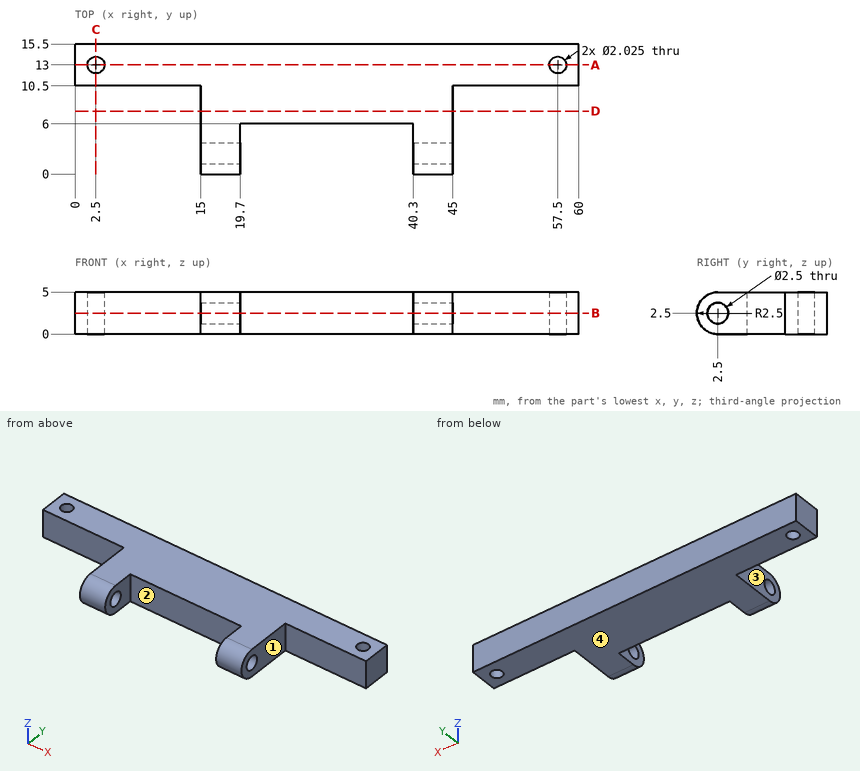
Could you check a few things on this drawing? It's one solid part, dimensions in mm from its lowest x, y, z. A direction names the side the tool comes from. Coordinates: 2 decimals unless noted, no trailing zeros. Order: outer loops, then holes, each group sorted by start corner. A loop starts at its lowest first (then second) coordinate and runs counter-clockwise, first axis right, second up.
1. If we section it at B-B (z = 2.5): Give the number of separate pieces and of enclosed holes in the cut face.
2. If we section it at A-A (y = 13): Please give me the cut outline in (x, z), then the cut area to 3 significant figures.
3. I'm going to push flat-ended pins straight in: pin 1 (3 mm diameter, centred on y = 7.5, z = 2.5, fed in from +X); pin 2 (3 mm diameter, centred on y = 8, z = 3, fed in from -X); pin 3 (1.5 mm diameter, centred on x = 10, z = 3, fed in from -Y); pin 4 (2.5 mm diameter, centred on x = 57.5, y = 13, fed in from +Z). Where does each tip first touch, or does it pass through?
4. For the marked faces 1, 2, 3 and 4, which set-ups out of +Z, -Z, +X, -X, +Y, -Y let a thin tool reach every point of the face, with its end or its side?
5. If we section it at D-D (y = 7.5): Please give me the cut outline in (x, z).
6. I need wall thicknesses on line 1 (X direction, y = 13, z = 1.25); line 2 (X direction, y = 5.5, z = 2.1); line 3 (Y direction, x = 42.55, z = 2.5). Which ranges of each line are inside material? Lowest first, please.
7. If we section it at C-C (x = 2.5): Please give me the cut outline in (y, z), then the cut area to 3 significant figures.
Entries:
1. separate pieces: 3
1. enclosed holes: 2
2. outline: (0, 0) - (1.49, 0) - (1.49, 5) - (0, 5) - close; (3.51, 0) - (56.49, 0) - (56.49, 5) - (3.51, 5) - close; (58.51, 0) - (60, 0) - (60, 5) - (58.51, 5) - close
2. area: 280 mm2
3. pin 1: stops at x = 45
3. pin 2: stops at x = 15
3. pin 3: stops at y = 10.5
3. pin 4: stops at z = 5
4. face 1: +Z, -Z, +X, -Y
4. face 2: +Z, -Z, -Y
4. face 3: +Z, -Z, -X, -Y
4. face 4: -Z, +X, -X, +Y, -Y
5. outline: (15, 0) - (45, 0) - (45, 5) - (15, 5) - close
6. line 1: x = 0 to 1.49, 3.51 to 56.49, 58.51 to 60
6. line 2: x = 15 to 19.7, 40.3 to 45
6. line 3: y = 0 to 1.25, 3.75 to 15.5
7. outline: (10.5, 0) - (11.99, 0) - (11.99, 5) - (10.5, 5) - close; (14.01, 0) - (15.5, 0) - (15.5, 5) - (14.01, 5) - close
7. area: 14.9 mm2
